```python
from build123d import *

# Parameters (mm, degrees)
F0_R     = 2.54
F1_DEPTH = 25.4
F2_T     = -2.54


with BuildPart() as f1:
    # F0 (on Top) → F1 (new body)
    with BuildSketch(Plane.XY):
        Polygon((184.18342, -10.24653), (-196.81658, -10.24653), (-171.41658, -35.64653), (158.78342, -35.64653), align=None)
        with Locations((-101.56658, -22.94653)):
            Circle(F0_R, mode=Mode.SUBTRACT)
        with Locations((-6.31658, -22.94653)):
            Circle(F0_R, mode=Mode.SUBTRACT)
        with Locations((88.93342, -22.94653)):
            Circle(F0_R, mode=Mode.SUBTRACT)
    extrude(amount=F1_DEPTH)

    # F2
    f2_openings = [f1.faces().sort_by_distance(p)[0] for p in [
        (-104.10658, -22.94653, 12.7),
        (-8.85658, -22.94653, 12.7),
        (86.39342, -22.94653, 12.7),
        (-184.11658, -22.94653, 12.7),
        (171.48342, -22.94653, 12.7),
        (-6.31658, -35.64653, 12.7),
        (168.783363, -20.246473, 25.4),
    ]]
    offset(amount=F2_T, openings=f2_openings)


solid = f1.part
```
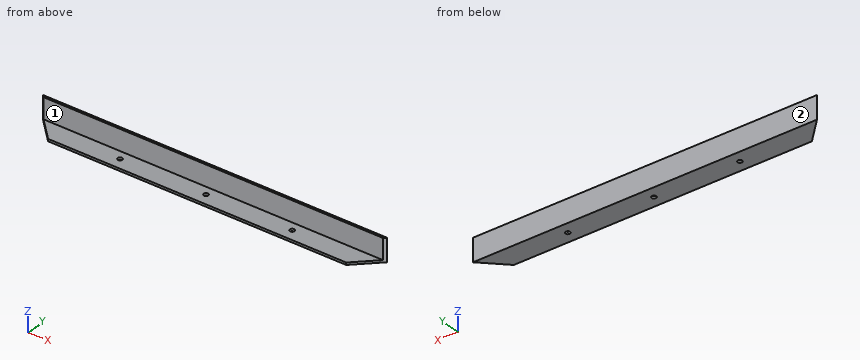
Geometry check sheet. Reference: the model listing, model coordinates, mm. Face numbers are marked on the shaded views. A direction names the side the tool comes from. Give positions to 0.01 mm unless a question says otherwise; leave off trailing zeros. Write each loop counter-clockwise with the first axis right and the second up, starting at its lowest first coordinate (ties: lowest second). Pieces come first, ordered by that corner, then holes. Notation, with made-up numbers: (84, 86.5) - (134, 86.5) arc R23 cw to (134, 125.5) - close; hole circle Ø11 at (25, 57.5). An arc over 180 degrees is marked (long way). Use a Markdown table: item, result.
Q1. Set-up check for the marked faces 1 and 2: record each of +Z, -Z, +X, -X, +Y, -Y from which the full face is reachable in a straight line by a thin tool's end or side.
Computed:
| item | result |
|---|---|
| face 1 | +Z, +X, -X, -Y |
| face 2 | +Z, -Z, +X, -X, +Y |
Q2. Section check A-A, the plane x = -33.5. Enter the section's corners in (y, z), then the cut area to 3 significant figures.
Computed:
| item | result |
|---|---|
| outline | (-35.65, 0) - (-10.25, 0) - (-10.25, 25.4) - (-12.79, 25.4) - (-12.79, 2.54) - (-35.65, 2.54) - close |
| area | 123 mm² |
Q3. Section check B-B, the plane z = 19. Enter the section's corners in (x, y).
Computed:
| item | result |
|---|---|
| outline | (-196.82, -10.25) - (-194.28, -12.79) - (181.64, -12.79) - (184.18, -10.25) - close |
Q4. Thickness scan on L1, parallel to Y at x = 127, z = 8.5; L2, parallel to Z at x = -167, y = -28.25; L3, parallel to Y at x = -100.5, z = 2.25. Record the ranges inside material, lowest first. Write a range as [from, to].
Computed:
| item | result |
|---|---|
| L1 | y = [-12.79, -10.25] |
| L2 | z = [0, 2.54] |
| L3 | y = [-35.65, -25.25], [-20.64, -10.25] |
Q5. Go/stop test with flat-tipped pins: P1, Ø1.5, axis at x = 60, y = -18.5, coming from the +Z side; P2, Ø11.5, axis at x = 27.5, z = 16.5, coming from the -Y side; P3, Ø8, axis at y = -18, z = 5.5, coming from the -X side. Record where each tip stops, or that it passes through.
Computed:
| item | result |
|---|---|
| P1 | stops at z = 2.54 |
| P2 | stops at y = -12.79 |
| P3 | stops at x = -191.75 |
Q6. Section check C-C, the plane y = -17. Enter the section's corners in (x, z), then the cut area to 3 significant figures.
Computed:
| item | result |
|---|---|
| outline | (-190.06, 0) - (177.43, 0) - (177.43, 2.54) - (-190.06, 2.54) - close |
| area | 933 mm² |
